Design review of the part built by this model. Coordinates are the model's own, in mm. A direction names the side the tool comes from. Round coordinates to 2 decimals unless told otherwise and drop trailing zeros. Order: outer loops, then holes, each group sorted by start corner. A loop starts at its lowest first (then second) coordinate and runs counter-clockwise, first axis right, second up. Notation, with made-up numbers: M 26.5,-2.5 L 74.5,-2.5 A13 ccw 74.5,14.5 Z; hole C 26.25,-38.5 d3. An arc over 180 degrees is marked long. Write each question's results on one line, items separated by ' | '. Start each with the question number.
Item 1: Clearance check with flat-ended pins moving along their axes: pin 1 (1.1 mm diameter, centred on x = 11, y = -36, fed in from -Z); pin 2 (11 mm diameter, centred on x = -1.5, y = 64, fed in from -Z) (3 decimals). State where each tip first meets the part, or that it passes through.
Item 2: Wall thickness on line 1 (Z direction, x = 1.5, y = 20); line 2 (Y direction, x = -5, z = -6); line 3 (Y direction, x = -6, z = -8.5): over which ranges is each line inside the solid? List them lowest first. Write a range as [from, to].
Item 3: Take a section at A-A, the plane z = -9. Write out the cut boundary in (x, y), plus the area to 3 significant figures.
Item 4: Take a section at C-C, the plane y = 27.5. Write out the cut boundary in (x, z).
Item 5: Machinability: for faces 1 (the flat face through (0, 12, -5)), 2 (the flat face through (0, 64, -5)), 3 (the flat face through (0, -36, -5)), which of the approach directions +Z, -Z, +X, -X, +Y, -Y give a long, thin tool a straight path to every point of the face, cutting with its end or side? Answer none if there is none.
Item 6: Take a section at B-B, the plane x = 13. Write out the cut boundary in (y, z), plus the area to 3 significant figures.
```python
from build123d import *

# Parameters (mm, degrees)
F1_DEPTH = 32


with BuildPart() as f1:
    # F0 (on Right) → F1 (new body, symmetric)
    with BuildSketch(Plane.YZ):
        with BuildLine():
            Line((-37.3383648694, 26.6163813695), (-37.3383648694, -5))
            Line((-37.3383648694, -5), (-33.6996619063, -5))
            ThreePointArc((-33.6996619063, -5), (-25.3498025253, 11.7240041235), (-10.7909497917, 0))
            ThreePointArc((-10.7909497917, 0), (-11.0669456682, -2.5588527336), (-11.882237677, -5))
            Line((-11.882237677, -5), (36.4290502083, -5))
            Line((36.4290502083, -5), (36.4290502083, 0))
            ThreePointArc((36.4290502083, 0), (48.4290502083, 12), (60.4290502083, 0))
            Line((60.4290502083, 0), (60.4290502083, -5))
            Line((60.4290502083, -5), (69.1487081349, -5))
            Line((69.1487081349, -5), (69.1487081349, 26.6163813695))
            Line((69.1487081349, 26.6163813695), (-37.3383648694, 26.6163813695))
        make_face()
        with BuildLine():
            Line((36.4290502083, 0), (36.4290502083, -5))
            Line((36.4290502083, -5), (37.5203380937, -5))
            ThreePointArc((37.5203380937, -5), (36.7050460848, -2.5588527336), (36.4290502083, 0))
        make_face()
        with BuildLine():
            ThreePointArc((-10.7909497917, 0), (-25.3498025253, 11.7240041235), (-33.6996619063, -5))
            Line((-33.6996619063, -5), (-11.882237677, -5))
            ThreePointArc((-11.882237677, -5), (-11.0669456682, -2.5588527336), (-10.7909497917, 0))
        make_face()
        with BuildLine():
            ThreePointArc((36.4290502083, 0), (36.7050460848, -2.5588527336), (37.5203380937, -5))
            Line((37.5203380937, -5), (59.337762323, -5))
            ThreePointArc((59.337762323, -5), (60.1530543318, -2.5588527336), (60.4290502083, 0))
            ThreePointArc((60.4290502083, 0), (48.4290502083, 12), (36.4290502083, 0))
        make_face()
        with BuildLine():
            Line((59.337762323, -5), (60.4290502083, -5))
            Line((60.4290502083, -5), (60.4290502083, 0))
            ThreePointArc((60.4290502083, 0), (60.1530543318, -2.5588527336), (59.337762323, -5))
        make_face()
        with BuildLine():
            Line((-11.882237677, -5), (-33.6996619063, -5))
            ThreePointArc((-33.6996619063, -5), (-22.7909497917, -12), (-11.882237677, -5))
        make_face()
        with BuildLine():
            Line((59.337762323, -5), (37.5203380937, -5))
            ThreePointArc((37.5203380937, -5), (48.4290502083, -12), (59.337762323, -5))
        make_face()
    extrude(amount=F1_DEPTH, both=True)


solid = f1.part
```
Results list:
1) pin 1: z = -5 | pin 2: z = -6.525
2) line 1: [-5, 26.62] | line 2: [-33.18, -12.4], [38.04, 58.82] | line 3: [-31.26, -14.32], [39.96, 56.9]
3) outline: M -32,-30.73 L 32,-30.73 L 32,-14.85 L -32,-14.85 Z; M -32,40.49 L 32,40.49 L 32,56.37 L -32,56.37 Z | area: 2,030 mm²
4) outline: M -32,-5 L 32,-5 L 32,26.62 L -32,26.62 Z
5) face 1: -Z, +X, -X | face 2: -Z, +X, -X, +Y | face 3: -Z, +X, -X, -Y
6) outline: M -37.34,-5 L -33.7,-5 A12 ccw -11.88,-5 L 37.52,-5 A12 ccw 59.34,-5 L 69.15,-5 L 69.15,26.62 L -37.34,26.62 Z | area: 3,590 mm²
